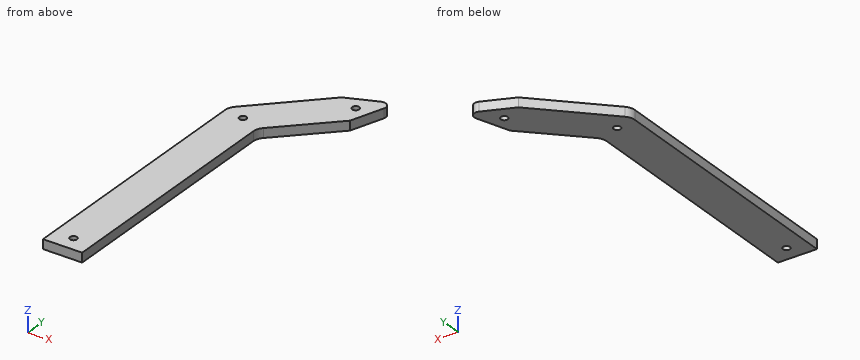
```python
from build123d import *

# Parameters (mm, degrees)
PAD_DEPTH    = 6
FILLET_R     = 8
FILLET001_R  = 8
FILLET002_R  = 4
SKETCH001_R  = 2.25
POCKET_DEPTH = 6


with BuildPart() as part:
    # Sketch → Pad (new body)
    with BuildSketch(Plane.XY):
        Polygon((0, 0), (25, 0), (25, 150), (25, 160), (60.104086, 194.748733), (70.142801, 223.906901), (42.426414, 212.4264), (0, 170), (0, 150), align=None)
    extrude(amount=PAD_DEPTH)

    # Fillet
    fillet_edges = [part.edges().sort_by_distance(p)[0] for p in [
        (0, 170, 3),
    ]]
    fillet(fillet_edges, radius=FILLET_R)

    # Fillet001
    fillet001_edges = [part.edges().sort_by_distance(p)[0] for p in [
        (25, 160, 3),
    ]]
    fillet(fillet001_edges, radius=FILLET001_R)

    # Fillet002
    fillet002_edges = [part.edges().sort_by_distance(p)[0] for p in [
        (70.142801, 223.906901, 3),
    ]]
    fillet(fillet002_edges, radius=FILLET002_R)

    # Sketch001 (on Face12 of Fillet002) → Pocket (cut)
    with BuildSketch(Plane.XY.offset(6)):
        with Locations((12.5, 165)):
            Circle(SKETCH001_R)
        with Locations((55, 207.25)):
            Circle(SKETCH001_R)
        with Locations((12.5, 10)):
            Circle(SKETCH001_R)
    extrude(amount=-POCKET_DEPTH, mode=Mode.SUBTRACT)


solid = part.part
```
The model under review builds one solid part; all positions refer to its coordinate system, in mm. Round coordinates to 2 decimals unless told otherwise and drop trailing zeros. Write each loop counter-clockwise with the first axis right and the second up, starting at its lowest first coordinate (ties: lowest second). Pieces come first, ordered by that corner, then holes. Notation, with made-up numbers: (68, -16.75) - (112, -16.75) arc R23 cw to (112, 12.25) - close; hole circle Ø4 at (-14.5, -15). An arc over 180 degrees is marked (long way). Answer as CSV lines item,"result". Start each with the question number.
(1) We need section A-A on x = 12.5. State the section outline as (y, z) points, plus the area to 3 significant figures.
(2) For pin 1 Ø5 at (x, y) = (23, 195) entering from +Z, flat-tipped, find the tip position at first contact; note if it passes through.
(3) We need section C-C on z = 1.55. State the section outline as (x, y) points, plus the area to 3 significant figures.
(4) We need section B-B on y = 10. State the section outline as (x, z) points.
(5) We need section D-D on x = 55. State the section outline as (y, z) points.
(6) To check wall thickness, follow line 1 (Y direction, x = 55, z = 4.3); line 2 (X direction, y = 147, z = 0.75); line 3 (Y direction, x = 56, z = 1.8). State the ranges of each line that lie inside material, in increasing order.
Worked answers:
1,outline,"(0, 0) - (7.75, 0) - (7.75, 6) - (0, 6) - close; (12.25, 0) - (162.75, 0) - (162.75, 6) - (12.25, 6) - close; (167.25, 0) - (182.5, 0) - (182.5, 6) - (167.25, 6) - close"
1,area,"1,040 mm²"
2,pin 1,"z = 6"
3,outline,"(0, 0) - (25, 0) - (25, 156.66) arc R8 cw to (27.37, 162.35) - (60.1, 194.75) - (67.25, 215.51) arc R4 ccw to (61.94, 220.51) - (42.43, 212.43) - (2.34, 172.34) arc R8 ccw to (0, 166.69) - close; hole circle Ø4.5 at (12.5, 10); hole circle Ø4.5 at (12.5, 165); hole circle Ø4.5 at (55, 207.25)"
3,area,"5,770 mm²"
4,outline,"(0, 0) - (10.25, 0) - (10.25, 6) - (0, 6) - close; (14.75, 0) - (25, 0) - (25, 6) - (14.75, 6) - close"
5,outline,"(189.7, 0) - (205, 0) - (205, 6) - (189.7, 6) - close; (209.5, 0) - (217.63, 0) - (217.63, 6) - (209.5, 6) - close"
6,line 1,"189.7 to 205, 209.5 to 217.63"
6,line 2,"0 to 25"
6,line 3,"190.69 to 205.23, 209.27 to 218.05"
